from build123d import *

# Parameters (mm, degrees)
ESQUISSE1_R        = 1.6
BOSS_EXTRU_1_DEPTH = 1.5


with BuildPart() as part:
    # Esquisse1 → Boss.-Extru.1 (new body)
    with BuildSketch(Plane.XY):
        Polygon((-75.988646329, 51.585106383), (42.975455994, 51.585106383), (51.669750275, 53.914735514), (147.250925797, 109.098552931), (210.540810955, 126.057026549), (216.43052053, 127.635169473), (224.324263617, 123.047292559), (225.851989006, 117.211223452), (230.508864659, 99.83152691), (241.906099495, 57.296467436), (237.335031683, 49.379145741), (178.515758799, 33.618569072), (73.963816863, -26.744522748), (63.997857106, -29.414893617), (-96.789296468, -29.414893617), (-103.253762562, -22.950427523), (-103.253762562, 35.79522772), (-103.253762562, 45.120640289), (-96.789296468, 51.585106383), align=None)
        with Locations((-95.753762562, 44.085106383)):
            Circle(ESQUISSE1_R, mode=Mode.SUBTRACT)
        with Locations((-66.988646329, 44.085106383)):
            Circle(ESQUISSE1_R, mode=Mode.SUBTRACT)
        with Locations((-95.753762562, -21.914893617)):
            Circle(ESQUISSE1_R, mode=Mode.SUBTRACT)
        with Locations((67.039694146, -20.835264486)):
            Circle(ESQUISSE1_R, mode=Mode.SUBTRACT)
        with Locations((49.263745973, 45.505477252)):
            Circle(ESQUISSE1_R, mode=Mode.SUBTRACT)
        with Locations((175.637377655, 40.567595866)):
            Circle(ESQUISSE1_R, mode=Mode.SUBTRACT)
        with Locations((150.12930694, 102.149526137)):
            Circle(ESQUISSE1_R, mode=Mode.SUBTRACT)
        with Locations((217.363403759, 120.120565138)):
            Circle(ESQUISSE1_R, mode=Mode.SUBTRACT)
        with Locations((234.393639901, 56.355573542)):
            Circle(ESQUISSE1_R, mode=Mode.SUBTRACT)
        Polygon((-93.253762562, 39.085106383), (-96.753762562, 39.085106383), (-96.753762562, 1.085106383), (-93.253762562, 1.085106383), (-93.253762562, -18.808291899), (-92.647160844, -19.414893617), (62.681332131, -19.414893617), (70.103960937, -17.426006223), (174.655902873, 42.937085598), (230.745845457, 57.966340417), (231.174777645, 58.70927276), (220.849606396, 97.243336459), (216.185262108, 114.650906326), (215.703467251, 116.491412548), (215.001377661, 116.899469991), (213.129001406, 116.397768286), (151.110781723, 99.780036406), (55.529606201, 44.596218989), (44.29198097, 41.585106383), (-75.988646329, 41.585106383), (-92.647160844, 41.585106383), (-93.253762562, 40.978504665), align=None, mode=Mode.SUBTRACT)
    extrude(amount=BOSS_EXTRU_1_DEPTH)


solid = part.part
Design review of the part built by this model. Coordinates are the model's own, in mm. A direction names the side the tool comes from. Coordinates: 2 decimals unless noted, no trailing zeros. Order: outer loops, then holes, each group sorted by start corner. A loop starts at its lowest first (then second) coordinate and runs counter-clockwise, first axis right, second up. Notation, with made-up numbers: M 61,-29.75 L 85,-29.75 A29 ccw 85,-4.75 Z; hole C 72.5,-4.75 d5. An arc over 180 degrees is marked long. Use a Markdown table: item, result.
(1) Add section B-B (y = 81). Give the boundary of the cut face in (x, z).
Worked answers:
| item | result |
|---|---|
| outline | M 98.58,0 L 118.58,0 L 118.58,1.5 L 98.58,1.5 Z; M 225.2,0 L 235.55,0 L 235.55,1.5 L 225.2,1.5 Z |
(2) For P1, Ø2.5, axis at x = -95.75, y = -21.91, coming from the +Z side; P2, Ø0.8, axis at y = 13, z = 0.5, coming from the +X side; P3, Ø0.8, axis at x = -28.5, z = 0.5, coming from the +Y side, all flat-tipped, find the tip position at first contact; note any pin that passes through.
Worked answers:
| item | result |
|---|---|
| P1 | passes through |
| P2 | stops at x = 143.5 |
| P3 | stops at y = 51.59 |
(3) For faces 1 (the flat face through (-99.976, -26.228, 0.74)), 2 (the flat face through (202.308, 50.347, 0.74)), list the 3-axis set-ups (+Z, -Z, +X, -X, +Y, -Y) from which the entire face can be reached by the end or side of a thin tool; tool diameter is ignored.
Worked answers:
| item | result |
|---|---|
| face 1 | +Z, -Z, -X, -Y |
| face 2 | +Z, -Z |
(4) Add section C-C (z = 0.95). Count the separate pieces of the cut face and the enclosed holes in it, then the cut area to 3 significant figures.
Worked answers:
| item | result |
|---|---|
| separate pieces | 1 |
| enclosed holes | 10 |
| area | 8,020 mm2 |
(5) Wall thickness on probe 1 along Y at (x, z) = (-34.5, 1.4); probe 2 along Y at (x, z) = (110, 0.45); probe 3 along X at (y, z) = (80, 1.3): over which ranges is each line inside the solid? List them lowest first.
Worked answers:
| item | result |
|---|---|
| probe 1 | y = -29.41 to -19.41, 41.59 to 51.59 |
| probe 2 | y = -5.94 to 5.61, 76.04 to 87.59 |
| probe 3 | x = 96.85 to 116.85, 225.47 to 235.82 |
(6) Add section A-A (x = -42). Give the boundary of the cut face in (y, z), then the cut area to 3 significant figures.
Worked answers:
| item | result |
|---|---|
| outline | M -29.41,0 L -19.41,0 L -19.41,1.5 L -29.41,1.5 Z; M 41.59,0 L 51.59,0 L 51.59,1.5 L 41.59,1.5 Z |
| area | 30.0 mm2 |
(7) Draft analysis for pull direction Y (two halves, no side actions). For faces 3 (the flat face through (208.3, 41.6, 0.7)), 4 (the flat face through (121.648, 12.333, 0.74)), 5 (the flat face through (-100.067, 48.308, 0.74)), 6 (the flat face through (70, 55, 1.5)), state which applies: released by +Y, released by -Y, zero draft, split by the parting line, or undercut.
Worked answers:
| item | result |
|---|---|
| face 3 | released by -Y |
| face 4 | undercut |
| face 5 | released by +Y |
| face 6 | zero draft |
